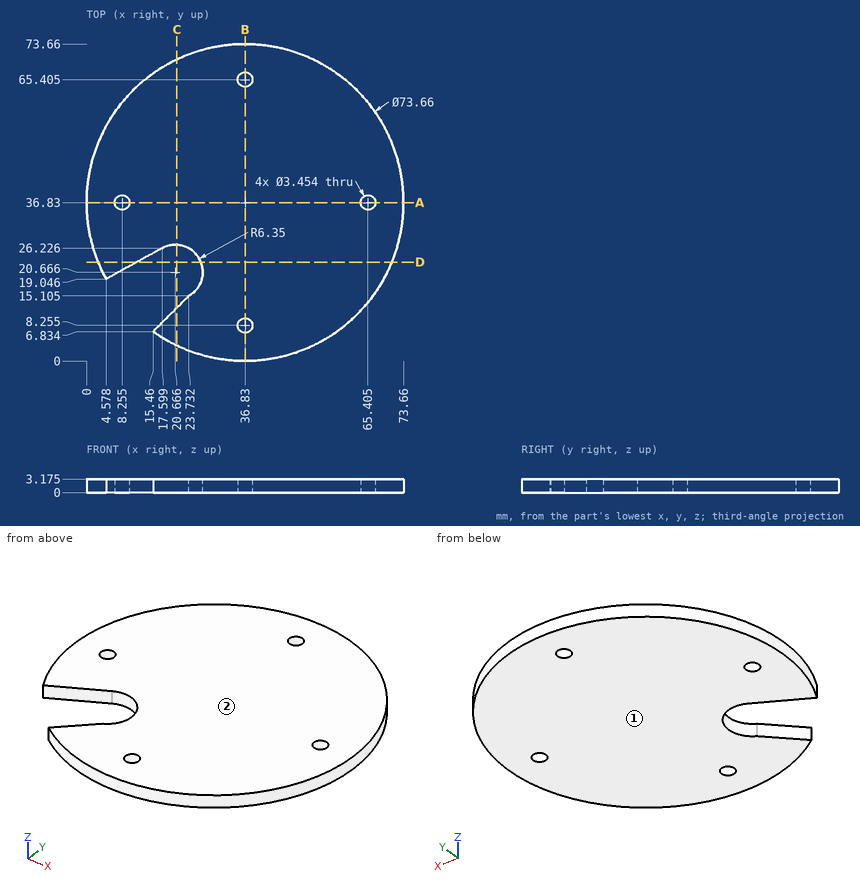
Can you work these out from the drawing? Everything is in mm from the part's minimum corner. Coordinates: 2 decimals unless noted, no trailing zeros. Loops run counter-clockwise (first coordinate to the right, second up) from the corner with the lowest first, then second, coordinate; pieces in that order, holes last.
1. Imagine slicing it at D-D, the plane y = 23. Please give me the cut outline in (x, z) (1 decimal).
2. Imagine slicing it at A-A, the plane y = 36.83. Please give me the cut outline in (x, z) (1 decimal), and give its area (3 significant figures).
3. For P1, Ø1.5, axis at x = 51.5, z = 2, coming from the +Y side; P2, Ø1.5, axis at x = 46, z = 1.5, coming from the +Y side (1 decimal), each with a flat end and sliding along its axis, tell me the tip position at first contact or that it passes through.
4. If we mould it in two halves opening along Z, with no side actions, what happens to the marked faces 1 and 2? For each: pulls with the +Z half, pulls with the -Z half, needs draft (parallel to the pull), parting line crosses it, or undercut.
5. I need wall thicknesses on L1, parallel to Y at x = 36.83, z = 1.15; L2, parallel to Y at x = 24, z = 1.9 (1 decimal); L3, parallel to X at y = 46.5, z = 2.35. Which ranges of each line are inside material? Lowest first, please.
6. Imagine slicing it at C-C, the plane x = 21. Please give me the cut outline in (y, z) (1 decimal).
Taken from the geometry:
1. outline: (2.7, 0) - (11.7, 0) - (11.7, 3.2) - (2.7, 3.2) - close; (26.6, 0) - (71, 0) - (71, 3.2) - (26.6, 3.2) - close
2. outline: (0, 0) - (6.5, 0) - (6.5, 3.2) - (0, 3.2) - close; (10, 0) - (63.7, 0) - (63.7, 3.2) - (10, 3.2) - close; (67.1, 0) - (73.7, 0) - (73.7, 3.2) - (67.1, 3.2) - close
2. area: 212 mm2
3. P1: stops at y = 70.93
3. P2: stops at y = 72.7
4. face 1: pulls with the -Z half
4. face 2: pulls with the +Z half
5. L1: y = 0 to 6.53, 9.98 to 63.68, 67.13 to 73.66
5. L2: y = 2.3 to 15.3, 26.1 to 71.4
5. L3: x = 1.29 to 72.37
6. outline: (3.6, 0) - (12.4, 0) - (12.4, 3.2) - (3.6, 3.2) - close; (27, 0) - (70.1, 0) - (70.1, 3.2) - (27, 3.2) - close
